Check sheet for the drawn part. Datum: minimum x, y, z corner. Units: mm. A direction names the side the tool comes from. Give positions to 0.01 mm unless a question says otherwise; leave off trailing zeros. Loops run counter-clockwise (first coordinate to the right, second up) from the corner with the lowest first, then second, coordinate; pieces in that order, holes last. Notation, with made-up numbers: (40.25, 32) - (46.25, 32) arc R14 ccw to (46.25, 48) - close; hole circle Ø10 at (59, -21.75). An arc over 180 degrees is marked (long way). Use one line per item in the form item = value.
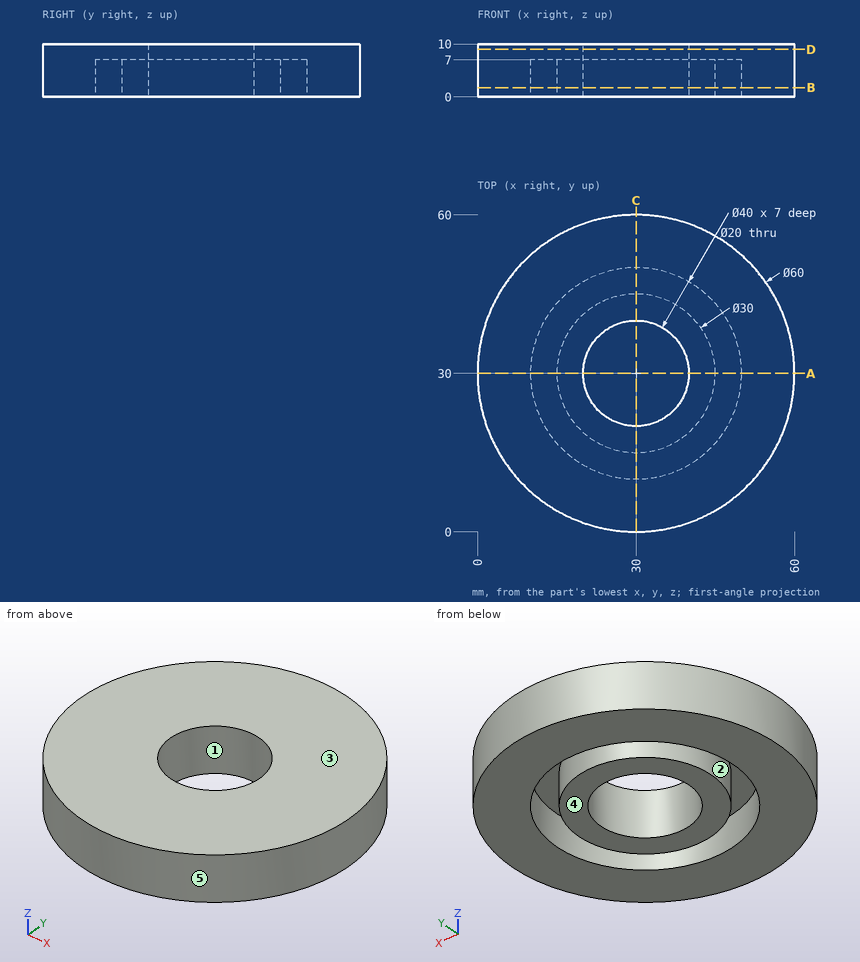
1. Depth check by flat-ended pin: pin 1 Ø2 at (y, z) = (15, 7) entering from -X; pin 2 Ø4 at (x, z) = (22, 1.5) entering from +Y; pin 3 Ø2 at (y, z) = (25.5, 5) entering from -X. Enter the tip coordinate at first touch or a pass-through.
Result set:
pin_1 = 3.47
pin_2 = 59.39
pin_3 = 0.2
2. Tool access check on the marked faces 1 and 2. Record the directions out of +Z, -Z, +X, -X, +Y, -Y that give a thin tool (end or side, any length) a straight path to the whole face; none if there is none.
Result set:
face_1 = +Z, -Z
face_2 = -Z
3. Section check B-B, the plane z = 1.75. Record the cut outline in (x, y).
Result set:
outline = circle Ø60 at (30, 30); circle Ø30 at (30, 30); hole circle Ø40 at (30, 30); hole circle Ø20 at (30, 30)
4. Draft check along Z on the marked faces 3, 4 and 5. Enter one of: released by +Z, released by -Z, zero draft, split by the parting line, or undercut.
Result set:
face_3 = released by +Z
face_4 = released by -Z
face_5 = zero draft
5. Section check D-D, the plane z = 9. Record the cut outline in (x, y).
Result set:
outline = circle Ø60 at (30, 30); hole circle Ø20 at (30, 30)
6. Section check A-A, the plane y = 30. Record the cut outline in (x, z).
Result set:
outline = (0, 0) - (10, 0) - (10, 7) - (15, 7) - (15, 0) - (20, 0) - (20, 10) - (0, 10) - close; (40, 0) - (45, 0) - (45, 7) - (50, 7) - (50, 0) - (60, 0) - (60, 10) - (40, 10) - close
7. Scan lines: probe 1 along Y at (x, z) = (29.5, 6); probe 2 along X at (y, z) = (22.5, 6); probe 3 along Y at (x, z) = (37, 3.75) (1 decimal). Record each from-to range of solid material in increasing order.
Result set:
probe_1 = 0 to 10.01, 15.01 to 20.01, 39.99 to 44.99, 49.99 to 60
probe_2 = 0.95 to 11.46, 17.01 to 23.39, 36.61 to 42.99, 48.54 to 59.05
probe_3 = 0.8 to 11.3, 16.7 to 22.9, 37.1 to 43.3, 48.7 to 59.2
